```python
from build123d import *

# Parameters (mm, degrees)
SKETCH1_W           = 70
SKETCH1_H           = 50
BOSS_EXTRUDE1_DEPTH = 5
SKETCH2_W           = 70
SKETCH2_H           = 7
BOSS_EXTRUDE2_DEPTH = 70
SKETCH3_R           = 2.1
SKETCH3_W           = 21
SKETCH3_H           = 41
CUT_EXTRUDE1_DEPTH  = 70
BOSS_EXTRUDE3_DEPTH = 5
BOSS_EXTRUDE4_DEPTH = 5
SKETCH8_R           = 2.1
CUT_EXTRUDE2_DEPTH  = 5
FILLET1_R           = 4
FILLET2_R           = 4


with BuildPart() as part:
    # Sketch1 → Boss-Extrude1 (new body)
    with BuildSketch(Plane(origin=(0, 0, 0), x_dir=(1, 0, 0), z_dir=(0, 1, 0))):
        Rectangle(SKETCH1_W, SKETCH1_H)
    extrude(amount=BOSS_EXTRUDE1_DEPTH)

    # Sketch2 → Boss-Extrude2 (add)
    with BuildSketch(Plane(origin=(0, 5, 0), x_dir=(1, 0, 0), z_dir=(0, 1, 0))):
        with Locations((0, 21.5)):
            Rectangle(SKETCH2_W, SKETCH2_H)
    extrude(amount=BOSS_EXTRUDE2_DEPTH)

    # Sketch3 → Cut-Extrude1 (cut)
    with BuildSketch(Plane(origin=(0, 0, -25), x_dir=(-1, 0, 0), z_dir=(0, 0, -1))):
        with Locations((-4.5, 65)):
            Circle(SKETCH3_R)
        with Locations((4.5, 65)):
            Circle(SKETCH3_R)
        with Locations((4.5, 14.7)):
            Circle(SKETCH3_R)
        with Locations((-4.5, 14.7)):
            Circle(SKETCH3_R)
        with Locations((0, 39.85)):
            Rectangle(SKETCH3_W, SKETCH3_H)
    extrude(amount=-CUT_EXTRUDE1_DEPTH, mode=Mode.SUBTRACT)

    # Sketch6 → Boss-Extrude3 (add)
    with BuildSketch(Plane.ZY.offset(35)):
        Polygon((-18, 75), (25, 5), (-18, 5), align=None)
    extrude(amount=-BOSS_EXTRUDE3_DEPTH)

    # Sketch7 → Boss-Extrude4 (add)
    with BuildSketch(Plane(origin=(35, 0, 0), x_dir=(0, 0, -1), z_dir=(1, 0, 0))):
        Polygon((18, 75), (-25, 5), (18, 5), align=None)
    extrude(amount=-BOSS_EXTRUDE4_DEPTH)

    # Sketch8 → Cut-Extrude2 (cut)
    with BuildSketch(Plane(origin=(0, 5, 0), x_dir=(1, 0, 0), z_dir=(0, 1, 0))):
        with Locations(Location((-16.347962706, 6, 0), (0, 0, 270))):
            Circle(SKETCH8_R)
        with Locations(Location((13.652037294, 6, 0), (0, 0, 270))):
            Circle(SKETCH8_R)
        with Locations(Location((-16.347962706, -19, 0), (0, 0, 270))):
            Circle(SKETCH8_R)
        with Locations(Location((13.652037294, -19, 0), (0, 0, 270))):
            Circle(SKETCH8_R)
    extrude(amount=-CUT_EXTRUDE2_DEPTH, mode=Mode.SUBTRACT)

    # Fillet1
    fillet1_edges = [part.edges().sort_by_distance(p)[0] for p in [
        (0, 5, -18),
    ]]
    fillet(fillet1_edges, radius=FILLET1_R)

    # Fillet2
    fillet2_edges = [part.edges().sort_by_distance(p)[0] for p in [
        (30, 42, -18),
        (30, 6.171572875, -16.828427125),
        (-30, 5, 5.5),
        (-30, 6.171572875, -16.828427125),
        (-30, 42, -18),
        (30, 5, 5.5),
    ]]
    fillet(fillet2_edges, radius=FILLET2_R)


solid = part.part
```
Input: part model. Units: mm. Frame: model coordinates. A direction names the side the tool comes from. Round coordinates to 2 decimals unless told otherwise and drop trailing zeros. Loops run counter-clockwise (first coordinate to the right, second up) from the corner with the lowest first, then second, coordinate; pieces in that order, holes last. Notation, with made-up numbers: M 45.5,70.5 L 72.5,70.5 A24 ccw 72.5,94.5 Z; hole C -24,77 d11. An arc over 180 degrees is marked long. Answer in a Markdown table with one row per item. Add a question column.
1. Section C-C (z = 19). Output: boundary loops of the cut face in (x, y).
2. Set-up query: faces 4 (the face through (0, 60.35, -22)), 5 (the face through (-35, 30, -5)), 6 (the face through (0.364, 6.203, -16.859)). Return all of +Z, -Z, +X, -X, +Y, -Y with unobstructed straight access to the full face (end or side cutting, diameter ignored); none if empty.
3. Contact query for flat-ended pins moving along their axis: pin 1 (2.5 mm diameter, centred on x = -16.35, z = 19, fed in from -Y); pin 2 (2 mm diameter, centred on x = -24.5, y = 48, fed in from +Z); pin 3 (8 mm diameter, centred on x = -9, z = -9.5, fed in from +Y). Output: stop coordinate, or through.
4. Section D-D (y = 66). Output: boundary loops of the cut face in (x, z).
5. Section A-A (x = 9). Output: boundary loops of the cut face in (y, z), and give its area (3 significant figures).
6. Mould query, pull axis Y, two halves, no side actions, for faces 1 (the face through (0, 19.35, -22)), 2 (the face through (32.56, 40.49, 3.2)), 3 (the face through (-12, 42, -18)). Classes: released by +Y, released by -Y, zero draft, split by the parting line, or undercut.
7. Ray query, probe 1 along X at (y, z) = (1.7, 19); probe 2 along Y at (x, z) = (4.5, -20.75); probe 3 along X at (y, z) = (58.5, -9.5). Return the intervals inside material, ascending.
8. Section B-B (y = 44). Output: boundary loops of the cut face in (x, z), and give its area (3 significant figures).
Values follow:
| question | item | result |
|---|---|---|
| 1 | outline | M -35,0 L -18.45,0 L -18.45,5 L -26,5 A4 cw -30,9 L -30,14.77 L -35,14.77 Z; M -14.25,0 L 11.55,0 L 11.55,5 L -14.25,5 Z; M 15.75,0 L 35,0 L 35,14.77 L 30,14.77 L 30,9 A4 cw 26,5 L 15.75,5 Z |
| 2 | face 4 | +Z, -Z |
| 2 | face 5 | +Z, -Z, -X, +Y, -Y |
| 2 | face 6 | +Z, +Y |
| 3 | pin 1 | through |
| 3 | pin 2 | z = -18 |
| 3 | pin 3 | y = 5 |
| 4 | outline | M -35,-25 L -6.35,-25 L -6.35,-18 L -26,-18 A4 cw -30,-14 L -30,-12.47 L -35,-12.47 Z; M -2.65,-25 L 2.65,-25 L 2.65,-18 L -2.65,-18 Z; M 6.35,-25 L 35,-25 L 35,-12.47 L 30,-12.47 L 30,-14 A4 cw 26,-18 L 6.35,-18 Z |
| 5 | outline | M 0,-25 L 19.35,-25 L 19.35,-18 L 9,-18 A4 cw 5,-14 L 5,25 L 0,25 Z; M 60.35,-25 L 75,-25 L 75,-18 L 60.35,-18 Z |
| 5 | area | 456 mm^2 |
| 6 | face 1 | undercut |
| 6 | face 2 | released by +Y |
| 6 | face 3 | zero draft |
| 7 | probe 1 | -35 to -18.45, -14.25 to 11.55, 15.75 to 35 |
| 7 | probe 2 | 0 to 12.6, 16.8 to 19.35, 60.35 to 62.9, 67.1 to 75 |
| 7 | probe 3 | -35 to -30, 30 to 35 |
| 8 | outline | M -35,-25 L -10.5,-25 L -10.5,-18 L -26,-18 A4 cw -30,-14 L -30,1.04 L -35,1.04 Z; M 10.5,-25 L 35,-25 L 35,1.04 L 30,1.04 L 30,-14 A4 cw 26,-18 L 10.5,-18 Z |
| 8 | area | 540 mm^2 |
